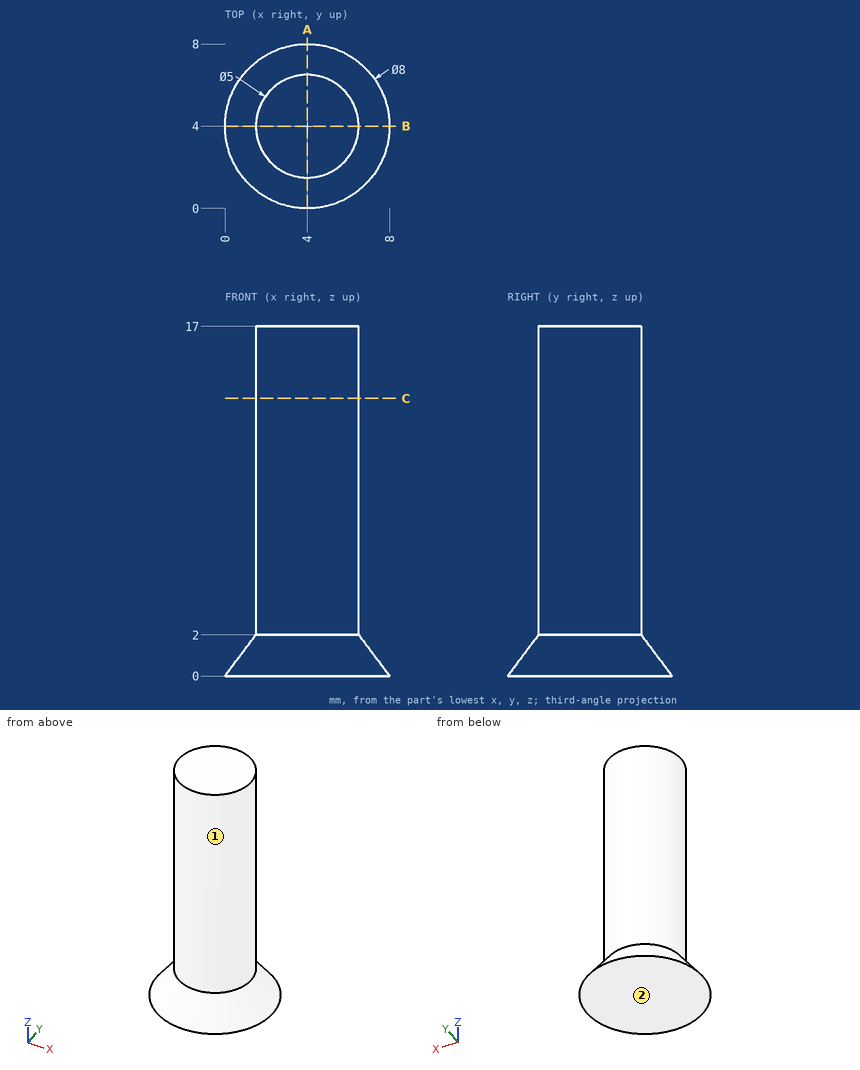
Job drawing, mm, ordinate dimensions from the low corner. One solid piece. A direction names the side the tool comes from. Give positions to 0.01 mm unless a question says otherwise; leave off trailing zeros. Loops run counter-clockwise (first coordinate to the right, second up) from the corner with the lowest first, then second, coordinate; pieces in that order, holes last. Notation, with made-up numbers: M 39,20 L 80,20 A14 ccw 80,41 Z; hole C 38.5,65.5 d6. An arc over 180 degrees is marked long. Put each result on its own line as item: value. Start each with the question number.
1) Flat gauge pins, fed straight in: pin 1 (1 mm diameter, centred on x = 6, y = 2, fed in from +Z); pin 2 (3 mm diameter, centred on x = 6, z = 5, fed in from -Y); pin 3 (1.5 mm diameter, centred on y = 2, z = 12, fed in from +X); pin 4 (4 mm diameter, centred on y = 1, z = 10, fed in from -X). Where does each tip first touch, or does it go through?
2) Saw through at A-A (x = 4). List the corners of the cut face in (y, z).
3) Probe probe 1 along Y at (x, z) = (5.5, 10.5); probe 2 along Z at (x, y) = (3.75, 6.75); probe 3 along Y at (x, z) = (4, 8). List the from-to ranges inside material, lowest first.
4) Saw through at C-C (z = 13.5). List the corners of the cut face in (x, y), then the cut area to 3 significant figures.
5) 3-axis set-ups, long thin cutter, end or side, ignore diameter. For the marked faces 1 and 2: which of +Z, -Z, +X, -X, +Y, -Y reach the whole face in a straight line?
Numbers:
1. pin 1: z = 17
1. pin 2: y = 1.55
1. pin 3: x = 6.17
1. pin 4: x = 1.71
2. outline: M 0,0 L 8,0 L 6.5,2 L 6.5,17 L 1.5,17 L 1.5,2 Z
3. probe 1: 2 to 6
3. probe 2: 0 to 1.65
3. probe 3: 1.5 to 6.5
4. outline: C 4,4 d5
4. area: 19.6 mm^2
5. face 1: +Z
5. face 2: -Z, +X, -X, +Y, -Y
